```python
from build123d import *

# Parameters (mm, degrees)
SKETCH_1_W          = 100
SKETCH_1_H          = 100
EXTRUDE_1_DEPTH     = 10
SKETCH_3_R          = 2.5
CUT_EXTRUDE_1_DEPTH = 10
SKETCH_3_3_R        = 1.5
CUT_EXTRUDE_2_DEPTH = 70
SKETCH_3_4_R        = 1.5
CUT_EXTRUDE_3_DEPTH = 70
SKETCH_3_7_R        = 2.5
CUT_EXTRUDE_4_DEPTH = 10
SKETCH_4_R          = 1
CUT_EXTRUDE_5_DEPTH = 5
SKETCH_2_R          = 2.65
CUT_EXTRUDE_6_DEPTH = 10
SKETCH_2_3_R        = 4.75
SKETCH_2_3_R_2      = 2.65
CUT_EXTRUDE_7_DEPTH = 5


with BuildPart() as part:
    # Sketch 1 → Extrude 1 (new body)
    with BuildSketch(Plane(origin=(0, 0, 0), x_dir=(1, 0, 0), z_dir=(0, 1, 0))):
        Rectangle(SKETCH_1_W, SKETCH_1_H)
    extrude(amount=EXTRUDE_1_DEPTH)

    # Sketch 3 → Cut-Extrude 1 (cut)
    with BuildSketch(Plane.XY.offset(50)):
        with Locations((-8, 5)):
            Circle(SKETCH_3_R)
    extrude(amount=-CUT_EXTRUDE_1_DEPTH, mode=Mode.SUBTRACT)

    # Sketch 3_3 → Cut-Extrude 2 (cut)
    with BuildSketch(Plane.XY.offset(50)):
        with Locations((-8, 5)):
            Circle(SKETCH_3_3_R)
    extrude(amount=-CUT_EXTRUDE_2_DEPTH, mode=Mode.SUBTRACT)

    # Sketch 3_4 → Cut-Extrude 3 (cut)
    with BuildSketch(Plane.XY.offset(50)):
        with Locations((8, 5)):
            Circle(SKETCH_3_4_R)
    extrude(amount=-CUT_EXTRUDE_3_DEPTH, mode=Mode.SUBTRACT)

    # Sketch 3_7 → Cut-Extrude 4 (cut)
    with BuildSketch(Plane.XY.offset(50)):
        with Locations((8, 5)):
            Circle(SKETCH_3_7_R)
    extrude(amount=-CUT_EXTRUDE_4_DEPTH, mode=Mode.SUBTRACT)

    # Sketch 4 → Cut-Extrude 5 (cut)
    with BuildSketch(Plane.XZ):
        with Locations(Location((-8.000069435, 35, 0), (0, 0, 270))):
            Circle(SKETCH_4_R)
        with Locations(Location((8, 35, 0), (0, 0, 270))):
            Circle(SKETCH_4_R)
        with Locations(Location((8, -16.5, 0), (0, 0, 270))):
            Circle(SKETCH_4_R)
        with Locations(Location((-8.000069435, -16.5, 0), (0, 0, 270))):
            Circle(SKETCH_4_R)
    extrude(amount=-CUT_EXTRUDE_5_DEPTH, mode=Mode.SUBTRACT)

    # Sketch 2 → Cut-Extrude 6 (cut)
    with BuildSketch(Plane(origin=(0, 10, 0), x_dir=(1, 0, 0), z_dir=(0, 1, 0))):
        with Locations(Location((0, 29, 0), (0, 0, 270))):
            Circle(SKETCH_2_R)
        with Locations(Location((0, 4, 0), (0, 0, 270))):
            Circle(SKETCH_2_R)
        with Locations(Location((-22, -35, 0), (0, 0, 270))):
            Circle(SKETCH_2_R)
        with Locations(Location((22, -35, 0), (0, 0, 270))):
            Circle(SKETCH_2_R)
    extrude(amount=-CUT_EXTRUDE_6_DEPTH, mode=Mode.SUBTRACT)

    # Sketch 2_3 → Cut-Extrude 7 (cut)
    # profile 1 of 4: a face of its own
    with BuildSketch(Plane(origin=(0, 10, 0), x_dir=(1, 0, 0), z_dir=(0, 1, 0))):
        with Locations(Location((-22, -35, 0), (0, 0, 270))):
            Circle(SKETCH_2_3_R)
        with Locations(Location((-22, -35, 0), (0, 0, 270))):
            Circle(SKETCH_2_3_R_2, mode=Mode.SUBTRACT)
    # profile 2 of 4: a face of its own
    with BuildSketch(Plane(origin=(0, 10, 0), x_dir=(1, 0, 0), z_dir=(0, 1, 0))):
        with Locations(Location((22, -35, 0), (0, 0, 270))):
            Circle(SKETCH_2_3_R)
        with Locations(Location((22, -35, 0), (0, 0, 270))):
            Circle(SKETCH_2_3_R_2, mode=Mode.SUBTRACT)
    # profile 3 of 4: a face of its own
    with BuildSketch(Plane(origin=(0, 10, 0), x_dir=(1, 0, 0), z_dir=(0, 1, 0))):
        with Locations(Location((0, 4, 0), (0, 0, 270))):
            Circle(SKETCH_2_3_R)
        with Locations(Location((0, 4, 0), (0, 0, 270))):
            Circle(SKETCH_2_3_R_2, mode=Mode.SUBTRACT)
    # profile 4 of 4: a face of its own
    with BuildSketch(Plane(origin=(0, 10, 0), x_dir=(1, 0, 0), z_dir=(0, 1, 0))):
        with Locations(Location((0, 29, 0), (0, 0, 270))):
            Circle(SKETCH_2_3_R)
        with Locations(Location((0, 29, 0), (0, 0, 270))):
            Circle(SKETCH_2_3_R_2, mode=Mode.SUBTRACT)
    extrude(amount=-CUT_EXTRUDE_7_DEPTH, mode=Mode.SUBTRACT)


solid = part.part
```
The model under review builds one solid part; all positions refer to its coordinate system, in mm. A direction names the side the tool comes from. Round coordinates to 2 decimals unless told otherwise and drop trailing zeros. Order: outer loops, then holes, each group sorted by start corner. A loop starts at its lowest first (then second) coordinate and runs counter-clockwise, first axis right, second up. Notation, with made-up numbers: (22, -23) -> (51, -23) arc R15 cw to (51, -6) -> close; hole circle Ø6 at (57.25, 51). An arc over 180 degrees is marked (long way). One line per item, written item: value. Start each with the question number.
Q1. Clearance check with flat-ended pins moving along their axes: pin 1 Ø3.5 at (x, y) = (-8.5, 5.5) entering from +Z; pin 2 Ø12.5 at (x, z) = (22, 35) entering from +Y; pin 3 Ø3 at (x, z) = (0, -29) entering from +Y; pin 4 Ø2.5 at (x, y) = (-8, 5) entering from +Z. State where each tip first meets the part, or that it passes through.
Q2. Machinability: for faces 1 (the face through (-1, 5, 50)), 2 (the face through (-8, 5, -20)), 3 (the face through (-1.819, 7.535, -24.612)), which of the approach directions +Z, -Z, +X, -X, +Y, -Y give a long, thin tool a straight path to every point of the face, cutting with its end or side? Answer none if there is none.
Q3. Take a section at B-B (z = -29). Write out the cut boundary in (x, y), and give its area (3 significant figures).
Q4. Mouldability with a two-part tool opening along Y and no side actions: class faces 4 (the face through (22.117, 2.535, 32.353)), 5 (the face through (-2, 5, -2)), 6 (the face through (10.385, 5.751, 45.07)) as released by +Y, released by -Y, zero draft, split by the parting line, or undercut.
Q5. Take a section at A-A (x = 0). Write out the cut boundary in (y, z), and give its area (3 significant figures).
Q6. Wall thickness on line 1 (X direction, y = 3, z = 41.5); line 2 (Z direction, x = 8, y = 3.1); line 3 (X direction, y = 8.4, z = 35): over which ranges is each line inside the solid? List them lowest first.
Reported:
1. pin 1: stops at z = 40
1. pin 2: stops at y = 10
1. pin 3: passes through
1. pin 4: stops at z = -20
2. face 1: +Z, +X, -X, +Y, -Y
2. face 2: +Z
2. face 3: +Y
3. outline: (-50, 0) -> (-2.65, 0) -> (-2.65, 5) -> (-4.75, 5) -> (-4.75, 10) -> (-50, 10) -> close; (2.65, 0) -> (50, 0) -> (50, 10) -> (4.75, 10) -> (4.75, 5) -> (2.65, 5) -> close
3. area: 926 mm2
4. face 4: zero draft
4. face 5: released by +Y
4. face 6: undercut
5. outline: (0, -50) -> (10, -50) -> (10, -33.75) -> (5, -33.75) -> (5, -31.65) -> (0, -31.65) -> close; (0, -26.35) -> (5, -26.35) -> (5, -24.25) -> (10, -24.25) -> (10, -8.75) -> (5, -8.75) -> (5, -6.65) -> (0, -6.65) -> close; (0, -1.35) -> (5, -1.35) -> (5, 0.75) -> (10, 0.75) -> (10, 50) -> (0, 50) -> close
5. area: 852 mm2
6. line 1: x = -50 to -9.5, -6.5 to 6.5, 9.5 to 50
6. line 2: z = -50 to -17.5, -15.5 to 34, 36 to 40
6. line 3: x = -50 to -26.75, -17.25 to 17.25, 26.75 to 50
